```python
from build123d import *

# Parameters (mm, degrees)
SKETCH1_W           = 410
SKETCH1_H           = 310
BOSS_EXTRUDE1_DEPTH = 1.5875
SKETCH2_R           = 3.175
SKETCH2_R_2         = 2
CUT_EXTRUDE1_DEPTH  = 258.006848462
SKETCH3_W           = 35
SKETCH3_H           = 15
CUT_EXTRUDE2_DEPTH  = 258.006848462


with BuildPart() as part:
    # Sketch1 → Boss-Extrude1 (new body)
    with BuildSketch(Plane(origin=(0, 0, 0), x_dir=(1, 0, 0), z_dir=(0, 1, 0))):
        Rectangle(SKETCH1_W, SKETCH1_H)
    extrude(amount=BOSS_EXTRUDE1_DEPTH)

    # Sketch2 → Cut-Extrude1 (cut, through all)
    with BuildSketch(Plane(origin=(0, 1.5875, 0), x_dir=(1, 0, 0), z_dir=(0, 1, 0))):
        with Locations(Location((-63.5, 127.06, 0), (0, 0, 270))):
            Circle(SKETCH2_R)
        with Locations(Location((-170, 120, 0), (0, 0, 270))):
            Circle(SKETCH2_R_2)
        with Locations(Location((63.5, 127.06, 0), (0, 0, 90))):
            Circle(SKETCH2_R)
        with Locations(Location((170, 120, 0), (0, 0, 90))):
            Circle(SKETCH2_R_2)
        with Locations(Location((170, -120, 0), (0, 0, 270))):
            Circle(SKETCH2_R_2)
        with Locations(Location((63.5, -127.06, 0), (0, 0, 270))):
            Circle(SKETCH2_R)
        with Locations(Location((-63.5, -127.06, 0), (0, 0, 90))):
            Circle(SKETCH2_R)
        with Locations(Location((-170, -120, 0), (0, 0, 90))):
            Circle(SKETCH2_R_2)
        with BuildLine():
            Line((-136.27, 155), (-133.73, 155))
            ThreePointArc((-133.73, 155), (-135, 153.73), (-136.27, 155))
        make_face()
        with BuildLine():
            Line((-86.27, 155), (-83.73, 155))
            ThreePointArc((-83.73, 155), (-85, 153.73), (-86.27, 155))
        make_face()
        with BuildLine():
            Line((86.27, 155), (83.73, 155))
            ThreePointArc((83.73, 155), (85, 153.73), (86.27, 155))
        make_face()
        with BuildLine():
            Line((136.27, 155), (133.73, 155))
            ThreePointArc((133.73, 155), (135, 153.73), (136.27, 155))
        make_face()
        with BuildLine():
            Line((136.27, -155), (133.73, -155))
            ThreePointArc((133.73, -155), (135, -153.73), (136.27, -155))
        make_face()
        with BuildLine():
            Line((86.27, -155), (83.73, -155))
            ThreePointArc((83.73, -155), (85, -153.73), (86.27, -155))
        make_face()
        with BuildLine():
            Line((-86.27, -155), (-83.73, -155))
            ThreePointArc((-83.73, -155), (-85, -153.73), (-86.27, -155))
        make_face()
        with BuildLine():
            Line((-136.27, -155), (-133.73, -155))
            ThreePointArc((-133.73, -155), (-135, -153.73), (-136.27, -155))
        make_face()
    extrude(amount=-CUT_EXTRUDE1_DEPTH, mode=Mode.SUBTRACT)

    # Sketch3 → Cut-Extrude2 (cut, through all)
    with BuildSketch(Plane(origin=(0, 1.5875, 0), x_dir=(1, 0, 0), z_dir=(0, 1, 0))):
        with Locations((-187.5, 147.5)):
            Rectangle(SKETCH3_W, SKETCH3_H)
        with Locations((187.5, -147.5)):
            Rectangle(SKETCH3_W, SKETCH3_H)
    extrude(amount=-CUT_EXTRUDE2_DEPTH, mode=Mode.SUBTRACT)


solid = part.part
```
CAD build for the part. Positions are in the model's coordinates, mm. Coordinates: 2 decimals unless noted, no trailing zeros. Write each loop counter-clockwise with the first axis right and the second up, starting at its lowest first coordinate (ties: lowest second). Pieces come first, ordered by that corner, then holes.
(1) Drill centre lines: probe 1 along X at (y, z) = (1.05, -127.06) (3 decimals); probe 2 along X at (y, z) = (1.1, -120); probe 3 along Z at (x, y) = (179, 0.8). Where is each one in solid material? Low to high.
(2) Flat gauge pins, fed straight in: pin 1 (0.8 mm diameter, centred on y = 0.5, z = -145, fed in from -X); pin 2 (0.5 mm diameter, centred on y = 0.5, z = 145.5, fed in from +X); pin 3 (4 mm diameter, centred on x = 63.5, z = -127.06, fed in from +Y); pin 4 (0.5 mm diameter, centred on x = 190.5, y = 1, fed in from +Z). Where does each tip first touch, or does it go through?
(3) Cut at A-A, the plane x = -177.5. List the corners of the cut face in (y, z), and give its area (3 significant figures).
Geometry says:
1. probe 1: x = -205 to -66.675, -60.325 to 60.325, 66.675 to 205
1. probe 2: x = -205 to -172, -168 to 168, 172 to 205
1. probe 3: z = -155 to 140
2. pin 1: stops at x = -170
2. pin 2: stops at x = 170
2. pin 3: passes through
2. pin 4: stops at z = 140
3. outline: (0, -140) - (1.59, -140) - (1.59, 155) - (0, 155) - close
3. area: 468 mm2
